Can you work these out from the drawing? Everything is in mm from the part's minimum corner. A direction names the side the tool comes from. Round coordinates to 2 decimals unless told otherwise and drop trailing zeros. Order: outer loops, then holes, each group sorted by start corner. A loop starts at its lowest first (then second) coordinate and runs counter-clockwise, first axis right, second up. Notation, with made-up numbers: M 20,67.5 L 44,67.5 A12 ccw 44,71.5 Z; hole C -39.75,36 d3. An arc over 180 degrees is marked long. Answer as CSV lines item,"result". Start each with the question number.
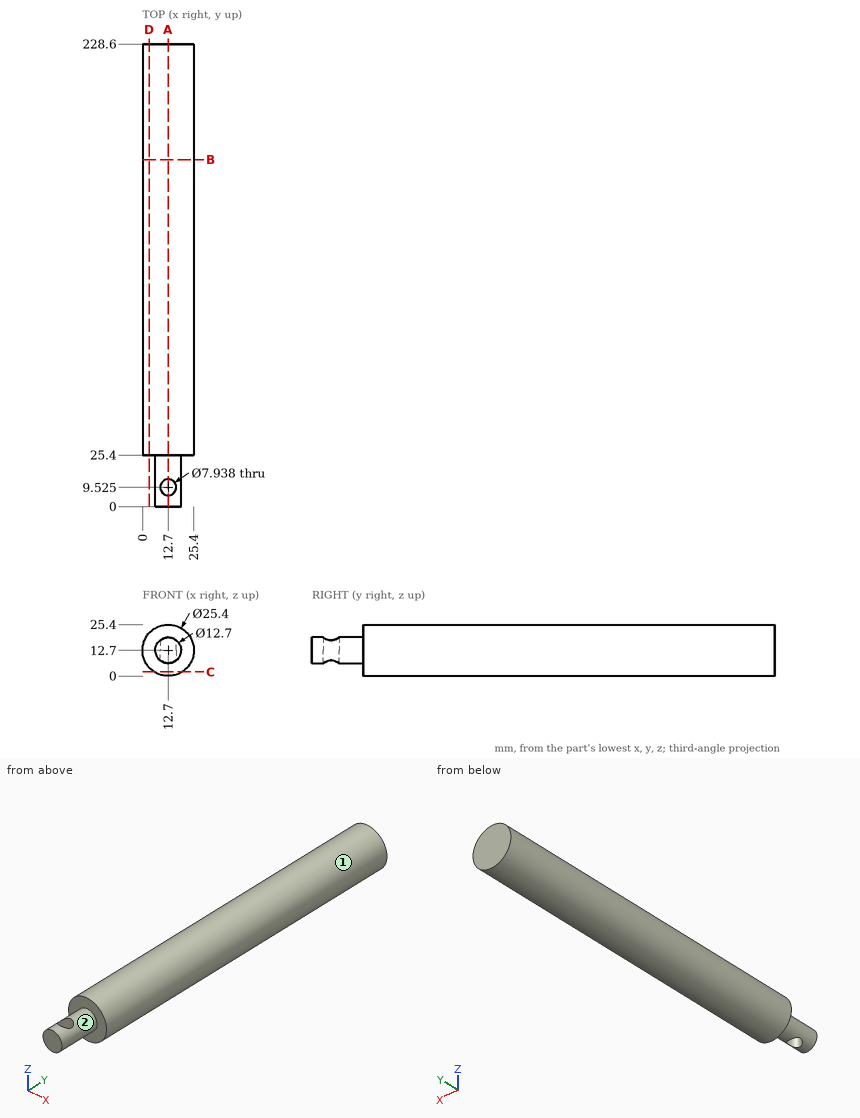
(1) I want a section at A-A on x = 12.7. Write out the boundary of the cut face in (y, z), and give its area (3 significant figures).
(2) If I drill on line 1 along Y through (x, z) = (12.7, 9.5); line 2 along Y through (x, z) = (23.25, 6.5); line 3 along X through (y, z) = (33, 11) (1 decimal), over which ranges is the centre line in solid material (lowest first)?
(3) I want a section at B-B on y = 171.5. Write out the boundary of the cut face in (x, z).
(4) I want a section at C-C on z = 2. Write out the boundary of the cut face in (x, y), and give its area (3 significant figures).
(5) I want a section at D-D on x = 3.25. Write out the boundary of the cut face in (y, z) (1 decimal).
(6) I'm going to push flat-ended pins straight in: P1, Ø4, axis at x = 3, y = 39.5, coming from the -Z side; P2, Ø5, axis at x = 7.5, y = 156.5, coming from the +Z side; P3, Ø9, axis at x = 12.7, y = 9.525, coming from the +Z side. Where does each tip first touch, or does it pass through?
(7) For the marked faces 1 and 2, which set-ups out of +Z, -Z, +X, -X, +Y, -Y let a thin tool reach every point of the face, with its end or its side?
From the geometry:
1,outline,"M 0,6.35 L 5.56,6.35 L 5.56,19.05 L 0,19.05 Z; M 13.49,6.35 L 25.4,6.35 L 25.4,0 L 228.6,0 L 228.6,25.4 L 25.4,25.4 L 25.4,19.05 L 13.49,19.05 Z"
1,area,"5,380 mm²"
2,line 1,"0 to 5.56, 13.49 to 228.6"
2,line 2,"25.4 to 228.6"
2,line 3,"0.1 to 25.3"
3,outline,"C 12.7,12.7 d25.4"
4,outline,"M 5.86,25.4 L 19.54,25.4 L 19.54,228.6 L 5.86,228.6 Z"
4,area,"2,780 mm²"
5,outline,"M 25.4,4.2 L 228.6,4.2 L 228.6,21.2 L 25.4,21.2 Z"
6,P1,"z = 2.6"
6,P2,"z = 25.11"
6,P3,"z = 19.05"
7,face 1,"+Y, -Y"
7,face 2,"-Y"
